from build123d import *

# Parameters (mm, degrees)
SKETCH1_W           = 152.4
SKETCH1_H           = 152.4
SKETCH1_R           = 3.175
BOSS_EXTRUDE1_DEPTH = 12
SKETCH2_W           = 12.0000014
SKETCH2_H           = 152.4
SKETCH2_W_2         = 3.076317806
SKETCH2_H_2         = 104.082085775
CUT_EXTRUDE1_DEPTH  = 3.175


with BuildPart() as part:
    # Sketch1 → Boss-Extrude1 (new body)
    with BuildSketch(Plane(origin=(0, 0, 0), x_dir=(1, 0, 0), z_dir=(0, 1, 0))):
        Rectangle(SKETCH1_W, SKETCH1_H)
        with Locations(Location((-50.8, 50.8, 0), (0, 0, 270))):
            Circle(SKETCH1_R, mode=Mode.SUBTRACT)
        with Locations(Location((50.8, 50.8, 0), (0, 0, 270))):
            Circle(SKETCH1_R, mode=Mode.SUBTRACT)
        with Locations(Location((-50.8, -50.8, 0), (0, 0, 270))):
            Circle(SKETCH1_R, mode=Mode.SUBTRACT)
        with Locations(Location((50.8, -50.8, 0), (0, 0, 270))):
            Circle(SKETCH1_R, mode=Mode.SUBTRACT)
    extrude(amount=BOSS_EXTRUDE1_DEPTH)

    # Sketch2 → Cut-Extrude1 (cut)
    with BuildSketch(Plane(origin=(0, 12, 0), x_dir=(1, 0, 0), z_dir=(0, 1, 0))):
        with Locations((-63.5, 0)):
            Rectangle(SKETCH2_W, SKETCH2_H)
        with Locations((-0.7000113, 0)):
            Rectangle(SKETCH2_W, SKETCH2_H)
        with Locations((35.270676847, 67.933500252)):
            Rectangle(SKETCH2_W_2, SKETCH2_H_2)
    extrude(amount=-CUT_EXTRUDE1_DEPTH, mode=Mode.SUBTRACT)


solid = part.part
Verification items for the finished model (mm, model axes). A direction names the side the tool comes from. Coordinates: 2 decimals unless noted, no trailing zeros. Order: outer loops, then holes, each group sorted by start corner. A loop starts at its lowest first (then second) coordinate and runs counter-clockwise, first axis right, second up. Notation, with made-up numbers: M 19.25,15 L 46.25,15 A35 cw 46.25,49 Z; hole C 23,59.25 d10. An arc over 180 degrees is marked long. One line per item, written item: value. Start each with the question number.
Item 1: Sectioned sample at B-B on z = -50.8. Record the cut outline in (x, y) (3 decimals).
Item 2: Sectioned sample at C-C on z = 65.5. Record the cut outline in (x, y) (3 decimals), then the cut area to 3 significant figures.
Item 3: Sectioned sample at D-D on z = -26. Record the cut outline in (x, y) (3 decimals).
Item 4: Mould release check, pull along Z, two halves, no side actions. Record for faces 3 (the cylindrical face through (-48.654, 5.916, -53.14)), 4 (the flat face through (-76.2, 6, 1)), 5 (the flat face through (-1, 6, 76.2)): pulls with the +Z half, pulls with the -Z half, needs draft (parallel to the pull), parting line crosses it, or undercut.
Item 5: Sectioned sample at A-A on x = -50.8. Record the cut outline in (y, z) (3 decimals).
Item 6: Thickness scan on probe 1 along X at (y, z) = (5.25, 50.8) (3 decimals); probe 2 along X at (y, z) = (10.75, 9); probe 3 along X at (y, z) = (9.5, 50.8) (3 decimals). Record the ranges inside material, lowest first.
Item 7: Depth check by flat-ended pin: P1, Ø4, axis at x = -50.8, z = 50.8, coming from the +Y side; P2, Ø3.5, axis at x = -63, z = -18, coming from the +Y side (3 decimals). Enter the tip coordinate at first touch or a pass-through.
Item 8: Access from +Z, -Z, +X, -X, +Y, -Y to the whole of each face (thin tool, end or side, straight path). Record for faces 1 (the flat face through (-64, 8.825, -1)), 2 (the flat face through (-1, 0, -1)).
Calculated:
1. outline: M -76.2,0 L -53.975,0 L -53.975,12 L -57.5,12 L -57.5,8.825 L -69.5,8.825 L -69.5,12 L -76.2,12 Z; M -47.625,0 L 47.625,0 L 47.625,12 L 36.809,12 L 36.809,8.825 L 33.733,8.825 L 33.733,12 L 5.3,12 L 5.3,8.825 L -6.7,8.825 L -6.7,12 L -47.625,12 Z; M 53.975,0 L 76.2,0 L 76.2,12 L 53.975,12 Z
2. outline: M -76.2,0 L 76.2,0 L 76.2,12 L 5.3,12 L 5.3,8.825 L -6.7,8.825 L -6.7,12 L -57.5,12 L -57.5,8.825 L -69.5,8.825 L -69.5,12 L -76.2,12 Z
2. area: 1,750 mm^2
3. outline: M -76.2,0 L 76.2,0 L 76.2,12 L 36.809,12 L 36.809,8.825 L 33.733,8.825 L 33.733,12 L 5.3,12 L 5.3,8.825 L -6.7,8.825 L -6.7,12 L -57.5,12 L -57.5,8.825 L -69.5,8.825 L -69.5,12 L -76.2,12 Z
4. face 3: undercut
4. face 4: needs draft
4. face 5: pulls with the +Z half
5. outline: M 0,-76.2 L 12,-76.2 L 12,-53.975 L 0,-53.975 Z; M 0,-47.625 L 12,-47.625 L 12,47.625 L 0,47.625 Z; M 0,53.975 L 12,53.975 L 12,76.2 L 0,76.2 Z
6. probe 1: -76.2 to -53.975, -47.625 to 47.625, 53.975 to 76.2
6. probe 2: -76.2 to -69.5, -57.5 to -6.7, 5.3 to 76.2
6. probe 3: -76.2 to -69.5, -57.5 to -53.975, -47.625 to -6.7, 5.3 to 47.625, 53.975 to 76.2
7. P1: through
7. P2: y = 8.825
8. face 1: +Z, -Z, +Y
8. face 2: +Z, -Z, +X, -X, -Y
